Verification items for the finished model (mm, model axes). Give positions to 0.01 mm unless a question says otherwise; leave off trailing zeros. Order: outer loops, then holes, each group sorted by start corner. A loop starts at its lowest first (then second) coordinate and runs counter-clockwise, first axis right, second up.
Autodesk Inventor part; units mm, degrees
ref_plane "YZ Plane" through (0, 0, 0) normal (1, 0, 0) x (0, 1, 0)
ref_plane "XZ Plane" through (0, 0, 0) normal (0, 1, 0) x (-1, 0, 0)
ref_plane "XY Plane" through (0, 0, 0) normal (0, 0, 1) x (1, 0, 0)
sketch "Sketch1" plane through (0, 0, 0) normal (0, 1, 0) x (-1, 0, 0)
  line L0 (9.525, 0) -> (66.675, 0)
  line L1 (76.2, -9.525) -> (76.2, -41.275)
  line L2 (66.675, -50.8) -> (9.525, -50.8)
  line L3 (0, -41.275) -> (0, -9.525)
  arc A0 (76.2, -9.525) -> (66.675, 0) centre (66.675, -9.525) ccw
  arc A1 (66.675, -50.8) -> (76.2, -41.275) centre (66.675, -41.275) ccw
  arc A2 (0, -41.275) -> (9.525, -50.8) centre (9.525, -41.275) ccw
  arc A3 (9.525, 0) -> (0, -9.525) centre (9.525, -9.525) ccw
  point P0 (0, 0)
  point P1 (76.2, 0)
  point P2 (76.2, -50.8)
  point P3 (0, -50.8)
  dimension "d0" = 50.8
  dimension "d1" = 76.2
  dimension "d2" = 9.525
  dimension "d3" = 9.525
extrude "Extrusion1" add sketch "Sketch1" along normal blind 2.54
properties part number "bottom ecoflex layer" material "PMMA Plastic"
(1) Scan lines: line 1 (Z direction, x = -3.5, y = 1.75); line 2 (X direction, y = 0.9, z = -42); line 3 (X direction, y = 0.3, z = -6.5). Record each from-to range of solid material in increasing order.
Solved:
line 1: z = -48.65 to -2.15
line 2: x = -76.17 to -0.03
line 3: x = -75.71 to -0.49
(2) Go/stop test with a flat-tipped pin: pin 1 (1.5 mm diameter, centred on x = -55.5, y = 1.5, fed in from +Z). Record where the tip stops, or that it passes through.
Solved:
pin 1: stops at z = 0
(3) Section check A-A, the plane y = 1.75. Enter the section's corners in (x, z) (3 decimals).
Solved:
outline: (-76.2, -41.275) arc R9.525 ccw to (-66.675, -50.8) - (-9.525, -50.8) arc R9.525 ccw to (0, -41.275) - (0, -9.525) arc R9.525 ccw to (-9.525, 0) - (-66.675, 0) arc R9.525 ccw to (-76.2, -9.525) - close
(4) Section check B-B, the plane z = -46. Enter the section's corners in (x, y), then the cut area to 3 significant figures.
Solved:
outline: (-74.95, 0) - (-1.25, 0) - (-1.25, 2.54) - (-74.95, 2.54) - close
area: 187 mm2
